Can you work these out from the model? Positions are in its coordinate system, mm. A direction names the side the tool comes from. Give positions to 0.01 mm unless a question says otherwise; leave off trailing zeros. Loops run counter-clockwise (first coordinate to the right, second up) from the corner with the lowest first, then second, coordinate; pieces in that order, holes last. Notation, with made-up numbers: (37, 4.25) -> (41, 4.25) arc R20 ccw to (41, 19.25) -> close; hole circle Ø8 at (-31.75, 39). An arc over 180 degrees is marked (long way). Return JSON: item names as keys, results as strings. Group by question number.
Q1. Suppose I cut it at A-A, the plane z = 335. Please give me the cut outline in (x, y).
Q2. Will these pins go through, and if not, where does the flat tip stop? pin 1 (5 mm diameter, centred on x = -7.5, z = 401.57, fed in from -Y); pin 2 (2.5 mm diameter, centred on x = -5, z = 105, fed in from +Y).
Q3. I need wall thicknesses on line 1 along X through (y, z) = (-13.85, 475); line 2 along Y through (x, z) = (5.5, 441.5). Which ranges of each line are inside material? Lowest first, please. Write a range as [from, to].
Q4. Suppose I cut it at B-B, the plane y = 3.75. Please give me the cut outline in (x, z).
Q5. Thinking about a two-plate mould opening in X: for faces 3 (the flat face through (-13, 0, 286)), 4 (the flat face through (0, 13, 286)), 5 (the flat face through (0, 15, 286)), 6 (the flat face through (-15, 0, 286)), which applies, pulls with the +X half, pulls with the -X half, needs draft (parallel to the pull), parting line crosses it, or undercut?
Q6. Which directions (+Z, -Z, +X, -X, +Y, -Y) give clear straight access to the entire face, cutting with the end or side of a thin tool? Please do faces 1 (the flat face through (15, 0, 286)), 2 (the flat face through (13, 0, 286)).
```python
from build123d import *

# Parameters (mm, degrees)
SKETCH_1_W          = 30
SKETCH_1_H          = 30
SKETCH_1_W_2        = 26
SKETCH_1_H_2        = 26
EXTRUDE_1_DEPTH     = 580
SKETCH_2_W          = 50
SKETCH_2_H          = 20
CUT_EXTRUDE_1_DEPTH = 581.969018107
SKETCH_3_R          = 2.1
CUT_EXTRUDE_2_DEPTH = 581.969018107
SKETCH_4_R          = 2.1
CUT_EXTRUDE_3_DEPTH = 581.969018107
SKETCH_7_R          = 2.1
CUT_EXTRUDE_4_DEPTH = 581.969018107


with BuildPart() as part:
    # 草图1 → 凸台-拉伸1 (new body)
    with BuildSketch(Plane.XY):
        Rectangle(SKETCH_1_W, SKETCH_1_H)
        Rectangle(SKETCH_1_W_2, SKETCH_1_H_2, mode=Mode.SUBTRACT)
    extrude(amount=EXTRUDE_1_DEPTH)

    # 草图2 → 切除-拉伸1 (cut, through all)
    with BuildSketch(Plane.ZY.offset(15)):
        with Locations((115, 0)):
            Rectangle(SKETCH_2_W, SKETCH_2_H)
        with Locations((465, 0)):
            Rectangle(SKETCH_2_W, SKETCH_2_H)
    extrude(amount=-CUT_EXTRUDE_1_DEPTH, mode=Mode.SUBTRACT)

    # 草图3 → 切除-拉伸2 (cut, through all)
    with BuildSketch(Plane(origin=(0, 15, 0), x_dir=(1, 0, 0), z_dir=(0, 1, 0))):
        with Locations(Location((7.5, -10, 0), (0, 0, 270))):
            Circle(SKETCH_3_R)
        with Locations(Location((-7.5, -10, 0), (0, 0, 270))):
            Circle(SKETCH_3_R)
        with Locations(Location((-7.5, -570, 0), (0, 0, 270))):
            Circle(SKETCH_3_R)
        with Locations(Location((7.5, -570, 0), (0, 0, 270))):
            Circle(SKETCH_3_R)
    extrude(amount=-CUT_EXTRUDE_2_DEPTH, mode=Mode.SUBTRACT)

    # 草图4 → 切除-拉伸3 (cut, through all)
    with BuildSketch(Plane(origin=(0, 15, 0), x_dir=(1, 0, 0), z_dir=(0, 1, 0))):
        with Locations(Location((7.5, -401.567476668, 0), (0, 0, 270))):
            Circle(SKETCH_4_R)
        with Locations(Location((-7.5, -401.567476668, 0), (0, 0, 270))):
            Circle(SKETCH_4_R)
        with Locations(Location((-7.5, -381.567476668, 0), (0, 0, 270))):
            Circle(SKETCH_4_R)
        with Locations(Location((7.5, -381.567476668, 0), (0, 0, 270))):
            Circle(SKETCH_4_R)
        with Locations(Location((7.5, -178.432523332, 0), (0, 0, 270))):
            Circle(SKETCH_4_R)
        with Locations(Location((-7.5, -178.432523332, 0), (0, 0, 270))):
            Circle(SKETCH_4_R)
        with Locations(Location((-7.5, -198.432523332, 0), (0, 0, 270))):
            Circle(SKETCH_4_R)
        with Locations(Location((7.5, -198.432523332, 0), (0, 0, 270))):
            Circle(SKETCH_4_R)
        with Locations((162.5, -178.432523332)):
            Circle(SKETCH_4_R)
        with Locations((177.5, -178.432523332)):
            Circle(SKETCH_4_R)
        with Locations((177.5, -198.432523332)):
            Circle(SKETCH_4_R)
        with Locations((162.5, -198.432523332)):
            Circle(SKETCH_4_R)
        with Locations((162.5, -381.567476668)):
            Circle(SKETCH_4_R)
        with Locations((162.5, -401.567476668)):
            Circle(SKETCH_4_R)
        with Locations((177.5, -401.567476668)):
            Circle(SKETCH_4_R)
        with Locations((177.5, -381.567476668)):
            Circle(SKETCH_4_R)
    extrude(amount=-CUT_EXTRUDE_3_DEPTH, mode=Mode.SUBTRACT)

    # 草图7 → 切除-拉伸4 (cut, through all)
    with BuildSketch(Plane(origin=(0, 15, 0), x_dir=(1, 0, 0), z_dir=(0, 1, 0))):
        with Locations(Location((5, -455, 0), (0, 0, 270))):
            Circle(SKETCH_7_R)
        with Locations(Location((-5, -455, 0), (0, 0, 270))):
            Circle(SKETCH_7_R)
        with Locations(Location((-5, -475, 0), (0, 0, 270))):
            Circle(SKETCH_7_R)
        with Locations(Location((5, -475, 0), (0, 0, 270))):
            Circle(SKETCH_7_R)
    cut_extrude_4 = extrude(amount=-CUT_EXTRUDE_4_DEPTH, mode=Mode.SUBTRACT)

    # 镜向1: 切除-拉伸4 across plane
    add(cut_extrude_4.mirror(Plane(origin=(0, 0, 290), x_dir=(1, 0, 0), z_dir=(0, 0, -1))), mode=Mode.SUBTRACT)


solid = part.part
```
Ans:
{
 "1": {"outline": "(-15, -15) -> (15, -15) -> (15, 15) -> (-15, 15) -> close; hole (-13, -13) -> (13, -13) -> (13, 13) -> (-13, 13) -> close"},
 "2": {"pin 1": "stops at y = -15", "pin 2": "passes through"},
 "3": {"line 1": "x = [-15, -7.1], [-2.9, 2.9], [7.1, 15]", "line 2": "y = [-15, -13], [13, 15]"},
 "4": {"outline": "(-15, 0) -> (-13, 0) -> (-13, 90) -> (-15, 90) -> close; (-15, 140) -> (-13, 140) -> (-13, 440) -> (-15, 440) -> close; (-15, 490) -> (-13, 490) -> (-13, 580) -> (-15, 580) -> close; (13, 0) -> (15, 0) -> (15, 90) -> (13, 90) -> close; (13, 140) -> (15, 140) -> (15, 440) -> (13, 440) -> close; (13, 490) -> (15, 490) -> (15, 580) -> (13, 580) -> close"},
 "5": {"face 3": "undercut", "face 4": "undercut", "face 5": "needs draft", "face 6": "pulls with the -X half"},
 "6": {"face 1": "+Z, -Z, +X, +Y, -Y", "face 2": "+Z, -Z"}
}
